Check sheet for the drawn part. Datum: minimum x, y, z corner. Units: mm. A direction names the side the tool comes from. Give positions to 0.01 mm unless a question says otherwise; leave off trailing zeros. Order: outer loops, then holes, each group sorted by start corner. A loop starts at its lowest first (then second) coordinate and runs counter-clockwise, first axis right, second up. Notation, with made-up numbers: (83, 67.5) -> (99, 67.5) arc R8 ccw to (99, 74.5) -> close; hole circle Ø9 at (49, 81). An arc over 180 degrees is marked (long way). One line per question, with ' | ' between items. Start each with the question number.
Q1. Section check B-B on x = 25.4. Record the cut outline in (y, z), plus the area to 3 significant figures.
Q2. Section check C-C on x = 32.5. Record the cut outline in (y, z), plus the area to 3 significant figures.
Q3. Section check D-D on x = 18. Record the cut outline in (y, z), plus the area to 3 significant figures.
Q4. Go/stop test with flat-tipped pins: pin 1 (1.5 mm diameter, centred on x = 28, z = 9, fed in from -Y); pin 2 (16 mm diameter, centred on x = 25.4, y = 30, fed in from +Z). Record where each tip stops, or that it passes through.
Q5. Access from +Z, -Z, +X, -X, +Y, -Y to the whole of each face (thin tool, end or side, straight path). Record for the marked faces 1 and 2.
Q6. Section check A-A on y = 30. Record the cut outline in (x, z), plus the area to 3 significant figures.
Q7. Material ranges on probe 1 along Y at (x, z) = (25.4, 8.8); probe 2 along Y at (x, z) = (25.4, 3.5); probe 3 along X at (y, z) = (30, 5.25), recorded low to high. Write a range as [from, to].
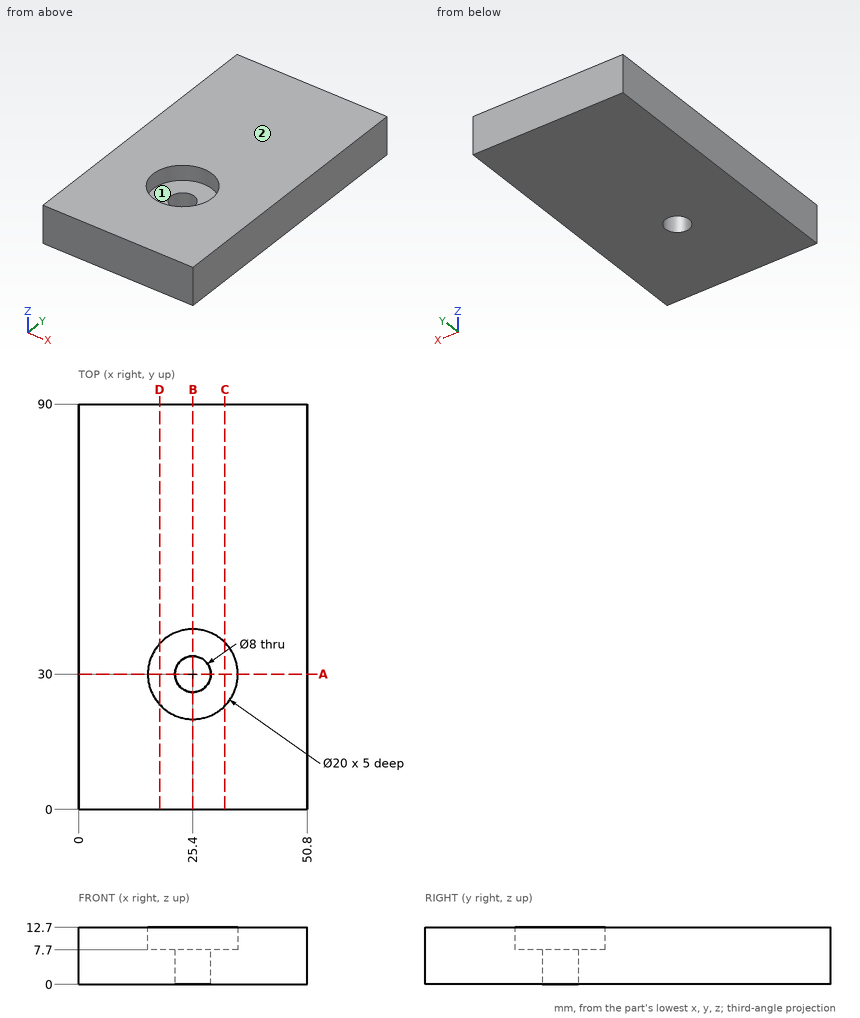
Filled in:
1) outline: (0, 0) -> (26, 0) -> (26, 7.7) -> (20, 7.7) -> (20, 12.7) -> (0, 12.7) -> close; (34, 0) -> (90, 0) -> (90, 12.7) -> (40, 12.7) -> (40, 7.7) -> (34, 7.7) -> close | area: 981 mm²
2) outline: (0, 0) -> (90, 0) -> (90, 12.7) -> (37.04, 12.7) -> (37.04, 7.7) -> (22.96, 7.7) -> (22.96, 12.7) -> (0, 12.7) -> close | area: 1,070 mm²
3) outline: (0, 0) -> (90, 0) -> (90, 12.7) -> (36.73, 12.7) -> (36.73, 7.7) -> (23.27, 7.7) -> (23.27, 12.7) -> (0, 12.7) -> close | area: 1,080 mm²
4) pin 1: y = 0 | pin 2: z = 7.7
5) face 1: +Z | face 2: +Z, +X, -X, +Y, -Y
6) outline: (0, 0) -> (21.4, 0) -> (21.4, 7.7) -> (15.4, 7.7) -> (15.4, 12.7) -> (0, 12.7) -> close; (29.4, 0) -> (50.8, 0) -> (50.8, 12.7) -> (35.4, 12.7) -> (35.4, 7.7) -> (29.4, 7.7) -> close | area: 484 mm²
7) probe 1: [0, 20], [40, 90] | probe 2: [0, 26], [34, 90] | probe 3: [0, 21.4], [29.4, 50.8]
